Geometry: final body of the model. Coordinates: model frame, mm. Face numbers are marked on the shaded views. Give positions to 0.01 mm unless a question says otherwise; leave off trailing zeros. Write each loop counter-clockwise with the first axis right and the second up, starting at its lowest first coordinate (ties: lowest second). Pieces come first, ordered by that corner, then holes.
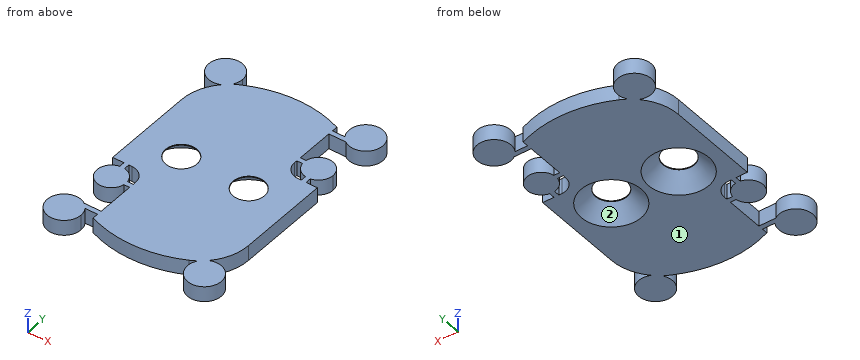
```python
from build123d import *

# Parameters (mm, degrees)
F0_R     = 3.25
F1_DEPTH = 3.175
F2_SIZE  = 3
F4_DEPTH = 3.175
F6_DEPTH = 3.175


with BuildPart() as f1:
    # F0 (on Top) → F1 (new body)
    with BuildSketch(Plane.XY):
        with BuildLine():
            Line((9, 10), (9, 21.7082933461))
            ThreePointArc((9, 21.7082933461), (-0.7933886028, 23.486603299), (-10.4444444444, 21.0514507872))
            ThreePointArc((-10.4444444444, 21.0514507872), (-14.498365856, 17.3638493894), (-16, 12.0933866224))
            Line((-16, 12.0933866224), (-16, -7))
            Line((-16, -7), (-12, -7))
            ThreePointArc((-12, -7), (-9.8786796564, -7.8786796564), (-9, -10))
            Line((-9, -10), (-9, -21.7082933461))
            ThreePointArc((-9, -21.7082933461), (0.7933886028, -23.486603299), (10.4444444444, -21.0514507872))
            ThreePointArc((10.4444444444, -21.0514507872), (14.498365856, -17.3638493894), (16, -12.0933866224))
            Line((16, -12.0933866224), (16, 7))
            Line((16, 7), (12, 7))
            ThreePointArc((12, 7), (9.8786796564, 7.8786796564), (9, 10))
        make_face()
        with Locations((-7, 0)):
            Circle(F0_R, mode=Mode.SUBTRACT)
        with Locations((7, 0)):
            Circle(F0_R, mode=Mode.SUBTRACT)
    extrude(amount=F1_DEPTH)

    # F2
    f2_edges = [f1.edges().sort_by_distance(p)[0] for p in [
        (-10.25, 0, 0),
        (3.75, 0, 0),
    ]]
    chamfer(f2_edges, length=F2_SIZE)

    # F3 (on face) → F4 (join, through all)
    with BuildSketch(Plane(origin=(0, 0, 0), x_dir=(1, 0, 0), z_dir=(0, 0, -1))):
        with BuildLine():
            ThreePointArc((-10.1919601085, 10.625), (-10.1605084316, 10.8741212192), (-10.15, 11.125))
            ThreePointArc((-10.15, 11.125), (-10.1605084316, 11.3758787808), (-10.1919601085, 11.625))
            Line((-10.1919601085, 11.625), (-12, 11.625))
            Line((-12, 11.625), (-12, 10.625))
            Line((-12, 10.625), (-10.1919601085, 10.625))
        make_face()
        with BuildLine():
            ThreePointArc((-10.1919601085, 11.625), (-10.1605084316, 11.3758787808), (-10.15, 11.125))
            ThreePointArc((-10.15, 11.125), (-10.1605084316, 10.8741212192), (-10.1919601085, 10.625))
            Line((-10.1919601085, 10.625), (-6, 10.625))
            Line((-6, 10.625), (-6, 11.625))
            Line((-6, 11.625), (-10.1919601085, 11.625))
        make_face()
        with BuildLine():
            Line((-12, 11.625), (-10.1919601085, 11.625))
            ThreePointArc((-10.1919601085, 11.625), (-15.2713203436, 13.2463203436), (-13.65, 8.1669601085))
            Line((-13.65, 8.1669601085), (-13.65, 10))
            Line((-13.65, 10), (-12.65, 10))
            Line((-12.65, 10), (-12.65, 8.1669601085))
            ThreePointArc((-12.65, 8.1669601085), (-11.0286796564, 9.0036796564), (-10.1919601085, 10.625))
            Line((-10.1919601085, 10.625), (-12, 10.625))
            Line((-12, 10.625), (-12, 11.625))
        make_face()
        with BuildLine():
            Line((-13.65, 10), (-13.65, 8.1669601085))
            ThreePointArc((-13.65, 8.1669601085), (-13.15, 8.125), (-12.65, 8.1669601085))
            Line((-12.65, 8.1669601085), (-12.65, 10))
            Line((-12.65, 10), (-13.65, 10))
        make_face()
        with BuildLine():
            ThreePointArc((-12.65, 8.1669601085), (-13.15, 8.125), (-13.65, 8.1669601085))
            Line((-13.65, 8.1669601085), (-13.65, 4))
            Line((-13.65, 4), (-12.65, 4))
            Line((-12.65, 4), (-12.65, 8.1669601085))
        make_face()
        with BuildLine():
            ThreePointArc((10.1919601085, -11.625), (13.4008787808, -14.1144915684), (16.15, -11.125))
            ThreePointArc((16.15, -11.125), (15.4412878475, -9.1885083269), (13.65, -8.1669601085))
            Line((13.65, -8.1669601085), (13.65, -10))
            Line((13.65, -10), (12.65, -10))
            Line((12.65, -10), (12.65, -8.1669601085))
            ThreePointArc((12.65, -8.1669601085), (11.0286796564, -9.0036796564), (10.1919601085, -10.625))
            Line((10.1919601085, -10.625), (12, -10.625))
            Line((12, -10.625), (12, -11.625))
            Line((12, -11.625), (10.1919601085, -11.625))
        make_face()
        with BuildLine():
            Line((13.65, -10), (13.65, -8.1669601085))
            ThreePointArc((13.65, -8.1669601085), (13.15, -8.125), (12.65, -8.1669601085))
            Line((12.65, -8.1669601085), (12.65, -10))
            Line((12.65, -10), (13.65, -10))
        make_face()
        with BuildLine():
            ThreePointArc((12.65, -8.1669601085), (13.15, -8.125), (13.65, -8.1669601085))
            Line((13.65, -8.1669601085), (13.65, -4))
            Line((13.65, -4), (12.65, -4))
            Line((12.65, -4), (12.65, -8.1669601085))
        make_face()
        with BuildLine():
            Line((6, -11.625), (10.1919601085, -11.625))
            ThreePointArc((10.1919601085, -11.625), (10.15, -11.125), (10.1919601085, -10.625))
            Line((10.1919601085, -10.625), (6, -10.625))
            Line((6, -10.625), (6, -11.625))
        make_face()
        with BuildLine():
            ThreePointArc((10.1919601085, -10.625), (10.15, -11.125), (10.1919601085, -11.625))
            Line((10.1919601085, -11.625), (12, -11.625))
            Line((12, -11.625), (12, -10.625))
            Line((12, -10.625), (10.1919601085, -10.625))
        make_face()
    extrude(amount=-F4_DEPTH)

    # F5 (on face) → F6 (join, through all)
    with BuildSketch(Plane(origin=(0, 0, 0), x_dir=(1, 0, 0), z_dir=(0, 0, -1))):
        with BuildLine():
            ThreePointArc((-11.5932314837, 20.5), (-11.2019974715, 21.3852645073), (-11.068175, 22.3438305439))
            ThreePointArc((-11.068175, 22.3438305439), (-17.6819252846, 23.9421293787), (-12.5279230945, 19.5))
            Line((-12.5279230945, 19.5), (-13.5525882542, 19.5))
            Line((-13.5525882542, 19.5), (-13.5525882542, 20.5))
            Line((-13.5525882542, 20.5), (-11.5932314837, 20.5))
        make_face()
        with BuildLine():
            Line((-13.5525882542, 19.5), (-12.5279230945, 19.5))
            ThreePointArc((-12.5279230945, 19.5), (-12.0112146406, 19.9538611465), (-11.5932314837, 20.5))
            Line((-11.5932314837, 20.5), (-13.5525882542, 20.5))
            Line((-13.5525882542, 20.5), (-13.5525882542, 19.5))
        make_face()
        with BuildLine():
            ThreePointArc((-11.5932314837, 20.5), (-12.0112146406, 19.9538611465), (-12.5279230945, 19.5))
            Line((-12.5279230945, 19.5), (-4.4474117458, 19.5))
            Line((-4.4474117458, 19.5), (-4.4474117458, 20.5))
            Line((-4.4474117458, 20.5), (-11.5932314837, 20.5))
        make_face()
        with BuildLine():
            ThreePointArc((-12.5279230945, -19.5), (-17.6819252846, -23.9421293787), (-11.068175, -22.3438305439))
            ThreePointArc((-11.068175, -22.3438305439), (-11.2019974715, -21.3852645073), (-11.5932314837, -20.5))
            Line((-11.5932314837, -20.5), (-13.5525882542, -20.5))
            Line((-13.5525882542, -20.5), (-13.5525882542, -19.5))
            Line((-13.5525882542, -19.5), (-12.5279230945, -19.5))
        make_face()
        with BuildLine():
            Line((-13.5525882542, -20.5), (-11.5932314837, -20.5))
            ThreePointArc((-11.5932314837, -20.5), (-12.0112146406, -19.9538611465), (-12.5279230945, -19.5))
            Line((-12.5279230945, -19.5), (-13.5525882542, -19.5))
            Line((-13.5525882542, -19.5), (-13.5525882542, -20.5))
        make_face()
        with BuildLine():
            ThreePointArc((-12.5279230945, -19.5), (-12.0112146406, -19.9538611465), (-11.5932314837, -20.5))
            Line((-11.5932314837, -20.5), (-4.4474117458, -20.5))
            Line((-4.4474117458, -20.5), (-4.4474117458, -19.5))
            Line((-4.4474117458, -19.5), (-12.5279230945, -19.5))
        make_face()
        with BuildLine():
            ThreePointArc((12.5279230945, 19.5), (16.1664738348, 19.2300802593), (18.068175, 22.3438305439))
            ThreePointArc((18.068175, 22.3438305439), (13.6096089635, 25.7100080724), (11.5932314837, 20.5))
            Line((11.5932314837, 20.5), (13.5525882542, 20.5))
            Line((13.5525882542, 20.5), (13.5525882542, 19.5))
            Line((13.5525882542, 19.5), (12.5279230945, 19.5))
        make_face()
        with BuildLine():
            Line((13.5525882542, 20.5), (11.5932314837, 20.5))
            ThreePointArc((11.5932314837, 20.5), (12.0112146406, 19.9538611465), (12.5279230945, 19.5))
            Line((12.5279230945, 19.5), (13.5525882542, 19.5))
            Line((13.5525882542, 19.5), (13.5525882542, 20.5))
        make_face()
        with BuildLine():
            ThreePointArc((12.5279230945, 19.5), (12.0112146406, 19.9538611465), (11.5932314837, 20.5))
            Line((11.5932314837, 20.5), (4.4474117458, 20.5))
            Line((4.4474117458, 20.5), (4.4474117458, 19.5))
            Line((4.4474117458, 19.5), (12.5279230945, 19.5))
        make_face()
        with BuildLine():
            ThreePointArc((11.5932314837, -20.5), (13.6096089635, -25.7100080724), (18.068175, -22.3438305439))
            ThreePointArc((18.068175, -22.3438305439), (16.1664738348, -19.2300802593), (12.5279230945, -19.5))
            Line((12.5279230945, -19.5), (13.5525882542, -19.5))
            Line((13.5525882542, -19.5), (13.5525882542, -20.5))
            Line((13.5525882542, -20.5), (11.5932314837, -20.5))
        make_face()
        with BuildLine():
            Line((13.5525882542, -19.5), (12.5279230945, -19.5))
            ThreePointArc((12.5279230945, -19.5), (12.0112146406, -19.9538611465), (11.5932314837, -20.5))
            Line((11.5932314837, -20.5), (13.5525882542, -20.5))
            Line((13.5525882542, -20.5), (13.5525882542, -19.5))
        make_face()
        with BuildLine():
            ThreePointArc((11.5932314837, -20.5), (12.0112146406, -19.9538611465), (12.5279230945, -19.5))
            Line((12.5279230945, -19.5), (4.4474117458, -19.5))
            Line((4.4474117458, -19.5), (4.4474117458, -20.5))
            Line((4.4474117458, -20.5), (11.5932314837, -20.5))
        make_face()
    extrude(amount=-F6_DEPTH)


solid = f1.part
```
Item 1: Pull-direction query (Y, two-part tool) for the marked faces 1 and 2; classes: +Y half, -Y half, draft (parallel to the pull), parting line (faces both ways), or undercut.
Found:
face 1: draft
face 2: undercut
Item 2: Section C-C, the plane z = 1.35. State how many separate pieces and enclosed holes the cut face has, plus the area to 3 significant figures.
Found:
separate pieces: 1
enclosed holes: 4
area: 1,260 mm2
Item 3: Pin query (flat end, axial travel): pin 1 Ø12 at (x, y) = (14.5, 13) entering from -Z; pin 2 Ø0.6 at (y, z) = (-21, 2) entering from -X; pin 3 Ø4 at (x, y) = (-7, 0) entering from -Z; pin 4 Ø1.6 at (y, z) = (-0.5, 1) entering from -X. Return the tip coordinate at first contact, or that it passes through.
Found:
pin 1: stops at z = 0
pin 2: stops at x = -17.91
pin 3: passes through
pin 4: stops at x = -16
Item 4: Section D-D, the plane y = 16. Return the cut outline in (x, z) (3 decimals).
Found:
outline: (-15.205, 0) - (9, 0) - (9, 3.175) - (-15.205, 3.175) - close
Item 5: Line query: L1, parallel to Y at x = 9.5, z = 0.55 (1 decimal); L2, parallel to X at y = -3, z = 1.15; L3, parallel to Y at x = 14, z = 1.8. Output: solid intervals per line, ascending.
Found:
L1: y = -21.5 to -5.1, 5.1 to 8.3, 10.6 to 11.6, 19.5 to 20.5
L2: x = -16 to -11.12, -2.88 to 2.88, 11.12 to 16
L3: y = -25.8 to -18.89, -18.09 to 7, 8.25 to 14, 18.89 to 25.8
Item 6: Section B-B, the plane x = -7. Return the cut outline in (y, z) (3 decimals).
Found:
outline: (-22.433, 0) - (-6.25, 0) - (-3.25, 3) - (-3.25, 3.175) - (-22.433, 3.175) - close; (3.25, 3) - (6.25, 0) - (22.433, 0) - (22.433, 3.175) - (3.25, 3.175) - close
Item 7: Section A-A, the plane y = 0. Return the cut outline in (x, z) (3 decimals), plus the area to 3 significant figures.
Found:
outline: (-16, 0) - (-13.25, 0) - (-10.25, 3) - (-10.25, 3.175) - (-16, 3.175) - close; (-3.75, 3) - (-0.75, 0) - (0.75, 0) - (3.75, 3) - (3.75, 3.175) - (-3.75, 3.175) - close; (10.25, 3) - (13.25, 0) - (16, 0) - (16, 3.175) - (10.25, 3.175) - close
area: 42.3 mm2
